```python
from build123d import *

# Parameters (mm, degrees)
SKETCH_1_R      = 2
SKETCH_1_R_2    = 5.280330007
EXTRUDE_1_DEPTH = 10
FILLET_1_R      = 1


with BuildPart() as part:
    # Эскиз1 → Бобышка-Вытянуть1 (new body)
    with BuildSketch(Plane(origin=(0, 0, 0), x_dir=(0, 0, -1), z_dir=(1, 0, 0))):
        Polygon((-5, 15.68), (-5, 10.68), (-5, 0), (-5, -5), (27, -5), (32, -5), (32, 15.68), align=None)
        Circle(SKETCH_1_R, mode=Mode.SUBTRACT)
        with Locations((27, 0)):
            Circle(SKETCH_1_R, mode=Mode.SUBTRACT)
        with Locations((0, 10.68)):
            Circle(SKETCH_1_R, mode=Mode.SUBTRACT)
        with Locations((13.5, 5.399669993)):
            Circle(SKETCH_1_R_2, mode=Mode.SUBTRACT)
        with Locations((27, 10.68)):
            Circle(SKETCH_1_R, mode=Mode.SUBTRACT)
    extrude(amount=EXTRUDE_1_DEPTH)

    # Скругление1
    fillet_1_edges = [part.edges().sort_by_distance(p)[0] for p in [
        (5, -5, -32),
        (5, -5, 5),
        (5, 15.68, 5),
        (5, 15.68, -32),
    ]]
    fillet(fillet_1_edges, radius=FILLET_1_R)


solid = part.part
```
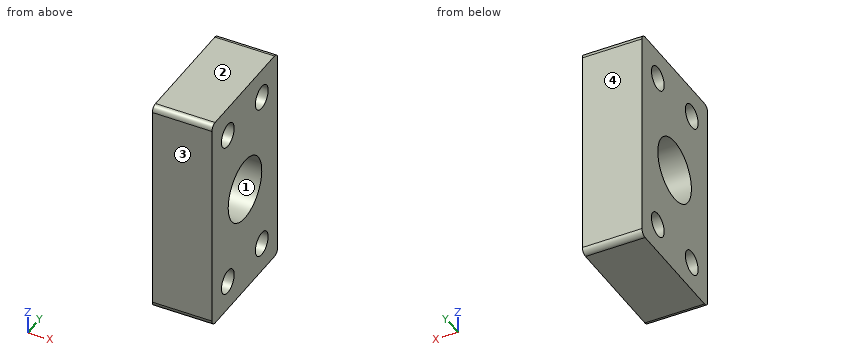
Input: part model. Units: mm. Frame: model coordinates. Face numbers are marked on the shaded views. Give positions to 0.01 mm unless a question says otherwise; leave off trailing zeros. Order: outer loops, then holes, each group sorted by start corner. A loop starts at its lowest first (then second) coordinate and runs counter-clockwise, first axis right, second up. Notation, with made-up numbers: (-10, -19.75) -> (25, -19.75) arc R17 ccw to (25, 4.25) -> close; hole circle Ø9 at (61, -21.5). An arc over 180 degrees is marked (long way). Write each question's results on one line, items separated by ' | '. Start each with the question number.
Item 1: Line query: line 1 (Y direction, x = 6.25, z = 0); line 2 (Y direction, x = 7.5, z = -1); line 3 (Z direction, x = 9, y = 10). Output: solid intervals per line, ascending.
Item 2: Cut plane B-B on z = 0. Return the cut outline in (x, y).
Item 3: Contact query for a flat-ended pin moving along its axis: P1, Ø3, axis at y = -1.5, z = -22.5, coming from the -X side. Output: stop coordinate, or through.
Item 4: Cut plane C-C on x = 8.75. Return the cut outline in (y, z), then the cut area to 3 significant figures.
Item 5: Mould query, pull axis Y, two halves, no side actions, for the marked faces 1, 2, 3 and 4. Classes: pulls with the +Y half, pulls with the -Y half, needs draft (parallel to the pull), parting line crosses it, or undercut.
Item 6: Cut plane D-D on y = 12.25. Return the cut outline in (x, z), then the cut area to 3 significant figures.
Item 7: Cut plane A-A on z = -13.5. Return the cut outline in (x, y).
Established:
1) line 1: -5 to -2, 2 to 8.68, 12.68 to 15.68 | line 2: -5 to -1.73, 1.73 to 8.95, 12.41 to 15.68 | line 3: -32 to -28.88, -25.12 to -16.09, -10.91 to -1.88, 1.88 to 5
2) outline: (0, -5) -> (10, -5) -> (10, -2) -> (0, -2) -> close; (0, 2) -> (10, 2) -> (10, 8.68) -> (0, 8.68) -> close; (0, 12.68) -> (10, 12.68) -> (10, 15.68) -> (0, 15.68) -> close
3) P1: x = 0
4) outline: (-5, -31) arc R1 ccw to (-4, -32) -> (14.68, -32) arc R1 ccw to (15.68, -31) -> (15.68, 4) arc R1 ccw to (14.68, 5) -> (-4, 5) arc R1 ccw to (-5, 4) -> close; hole circle Ø4 at (0, -27); hole circle Ø4 at (0, 0); hole circle Ø10.56 at (5.4, -13.5); hole circle Ø4 at (10.68, -27); hole circle Ø4 at (10.68, 0) | area: 626 mm^2
5) face 1: undercut | face 2: needs draft | face 3: pulls with the -Y half | face 4: pulls with the +Y half
6) outline: (0, -32) -> (10, -32) -> (10, -28.24) -> (0, -28.24) -> close; (0, -25.76) -> (10, -25.76) -> (10, -1.24) -> (0, -1.24) -> close; (0, 1.24) -> (10, 1.24) -> (10, 5) -> (0, 5) -> close | area: 320 mm^2
7) outline: (0, -5) -> (10, -5) -> (10, 0.12) -> (0, 0.12) -> close; (0, 10.68) -> (10, 10.68) -> (10, 15.68) -> (0, 15.68) -> close
